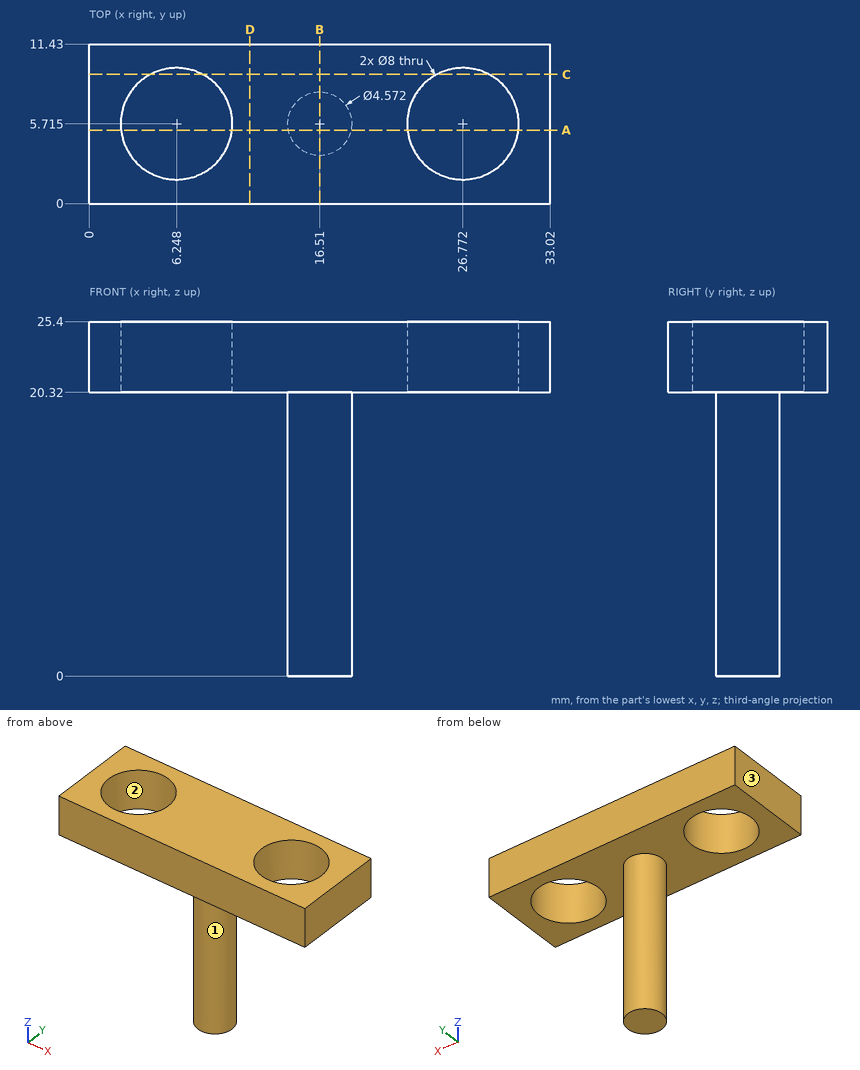
Design review of the part shown in the three views and the two pictorial views. Dimensions are in mm from the part's minimum x, y and z. Round coordinates to 2 decimals unless told otherwise and drop trailing zeros. Write each loop counter-clockwise with the first axis right and the second up, starting at its lowest first coordinate (ties: lowest second). Pieces come first, ordered by that corner, then holes.
Item 1: Draft analysis for pull direction Y (two halves, no side actions). For the marked faces 1, 2 and 3, state which applies: released by +Y, released by -Y, zero draft, split by the parting line, or undercut.
Item 2: Consider section A-A on y = 5.25. Give the boundary of the cut face in (x, z) (1 decimal).
Item 3: Consider section C-C on y = 9.25. Give the boundary of the cut face in (x, z), and give its area (3 significant figures).
Item 4: For pin 1 Ø4 at (x, y) = (22.5, 7) entering from -Z; pin 2 Ø4 at (y, z) = (2, 22) entering from -X; pin 3 Ø8 at (x, z) = (18, 8) entering from -Y; pin 4 Ø6 at (y, z) = (5, 7.5) entering from -X, all flat-tipped, find the tip position at first contact; note any pin that passes through.
Item 5: Wall thickness on L1, parallel to X at y = 3, z = 23.5 (1 decimal); L2, parallel to Z at x = 20, y = 10; L3, parallel to Y at x = 15, z = 19.25: over which ranges is each line inside the solid? List them lowest first.
Item 6: Consider section B-B on x = 16.51. Give the boundary of the cut face in (y, z).
Item 7: Consider section D-D on x = 11.5. Give the boundary of the cut face in (y, z).
Check values:
1. face 1: split by the parting line
1. face 2: undercut
1. face 3: zero draft
2. outline: (0, 20.3) - (2.3, 20.3) - (2.3, 25.4) - (0, 25.4) - close; (10.2, 20.3) - (14.3, 20.3) - (14.3, 0) - (18.7, 0) - (18.7, 20.3) - (22.8, 20.3) - (22.8, 25.4) - (10.2, 25.4) - close; (30.7, 20.3) - (33, 20.3) - (33, 25.4) - (30.7, 25.4) - close
3. outline: (0, 20.32) - (4.38, 20.32) - (4.38, 25.4) - (0, 25.4) - close; (8.12, 20.32) - (24.9, 20.32) - (24.9, 25.4) - (8.12, 25.4) - close; (28.64, 20.32) - (33.02, 20.32) - (33.02, 25.4) - (28.64, 25.4) - close
3. area: 130 mm2
4. pin 1: stops at z = 20.32
4. pin 2: stops at x = 0
4. pin 3: stops at y = 3.43
4. pin 4: stops at x = 14.22
5. L1: x = 0 to 3.3, 9.2 to 23.8, 29.7 to 33
5. L2: z = 20.32 to 25.4
5. L3: y = 4 to 7.43
6. outline: (0, 20.32) - (3.43, 20.32) - (3.43, 0) - (8, 0) - (8, 20.32) - (11.43, 20.32) - (11.43, 25.4) - (0, 25.4) - close
7. outline: (0, 20.32) - (11.43, 20.32) - (11.43, 25.4) - (0, 25.4) - close
